Source: CAD feature listing. Evaluate the final solid. Frame: model axes, mm. Face numbers are marked on the shaded views. A direction names the side the tool comes from. Give positions to 0.01 mm unless a question says otherwise; leave off trailing zeros. Write each loop counter-clockwise with the first axis right and the second up, starting at its lowest first coordinate (ties: lowest second). Pieces come first, ordered by that corner, then holes. Notation, with made-up numbers: (48, 62.25) -> (71, 62.25) arc R12 ccw to (71, 72.25) -> close; hole circle Ø10 at (39, 20). An arc over 180 degrees is marked (long way). Answer as a JSON object with one key per item and string values. Group by question number.
Item 1: Section query B-B on z = 0. Return the cut outline in (x, y).
Item 2: Ray query, probe 1 along Y at (x, z) = (1.5, 7.5); probe 2 along X at (y, z) = (-24, -0.25); probe 3 along Z at (x, y) = (-0.5, 11). Return the intervals inside material, ascending. Write a range as from..to.
Item 3: Section query D-D on x = 8.25. Return the cut outline in (y, z).
Item 4: First-contact query: pin 1 Ø5 at (y, z) = (50, -6.5) entering from -X; pin 2 Ø6 at (y, z) = (43, -3) entering from -X; pin 3 Ø8 at (y, z) = (1.5, 3.5) entering from -X; pin 4 Ø1.5 at (x, z) = (6, 7) entering from +Y. Flat tips, straight axial feed; report the tip coordinate or a pass-through.
Item 5: Access query for the marked faces 1, 2 and 3. Directions: +Z, -Z, +X, -X, +Y, -Y. A direction counts if a zero-diameter tool reaches every point of the face in a straight line with its end or side. Return the directions, or none.
Item 6: Section query A-A on x = 0. Return the cut outline in (y, z), plus the area to 3 significant figures.
Item 7: Section query C-C on y = 11. Return the cut outline in (x, z).
from build123d import *

# Parameters (mm, degrees)
BOSS_EXTRUDE1_DEPTH      = 65
BOSS_EXTRUDE1_DEPTH_BACK = 34
SKETCH1_R                = 7
SKETCH2_R                = 9.5
BOSS_EXTRUDE2_DEPTH      = 3


with BuildPart() as part:
    # Sketch1 → Boss-Extrude1 (new, two sides: drawn at the far end of the back side and taken through both)
    with BuildSketch(Plane(origin=(0, 0, 0), x_dir=(1, 0, 0), z_dir=(0, 1, 0)).offset(-BOSS_EXTRUDE1_DEPTH_BACK)):
        with Locations(Location((0, 0, 0), (0, 0, 270))):
            Circle(SKETCH1_R)
    extrude(amount=BOSS_EXTRUDE1_DEPTH + BOSS_EXTRUDE1_DEPTH_BACK)

    # Sketch2 → Boss-Extrude2 (add)
    with BuildSketch(Plane(origin=(0, 0, 0), x_dir=(1, 0, 0), z_dir=(0, 1, 0))):
        with Locations(Location((0, 0, 0), (0, 0, 270))):
            Circle(SKETCH2_R)
    extrude(amount=-BOSS_EXTRUDE2_DEPTH)


solid = part.part
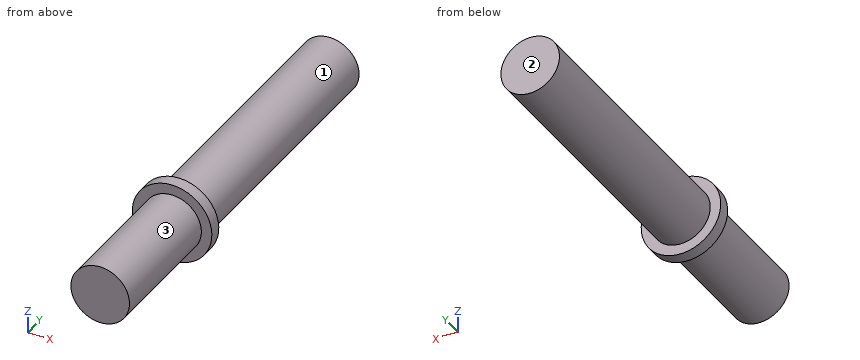
Worked answers:
{
 "1": {"outline": "(-9.5, -3) -> (-7, -3) -> (-7, -34) -> (7, -34) -> (7, -3) -> (9.5, -3) -> (9.5, 0) -> (7, 0) -> (7, 65) -> (-7, 65) -> (-7, 0) -> (-9.5, 0) -> close"},
 "2": {"probe 1": "-3..0", "probe 2": "-7..7", "probe 3": "-6.98..6.98"},
 "3": {"outline": "(-3, -4.71) -> (0, -4.71) -> (0, 4.71) -> (-3, 4.71) -> close"},
 "4": {"pin 1": "x = -5.74", "pin 2": "x = -7", "pin 3": "x = -9.5", "pin 4": "y = 0"},
 "5": {"face 1": "+Y", "face 2": "+Z, -Z, +X, -X, +Y", "face 3": "-Y"},
 "6": {"outline": "(-34, -7) -> (-3, -7) -> (-3, -9.5) -> (0, -9.5) -> (0, -7) -> (65, -7) -> (65, 7) -> (0, 7) -> (0, 9.5) -> (-3, 9.5) -> (-3, 7) -> (-34, 7) -> close", "area": "1,400 mm^2"},
 "7": {"outline": "circle Ø14 at (0, 0)"}
}
